Check sheet for the modelled part. Datum: model origin and axes. Units: mm. A direction names the side the tool comes from. Round coordinates to 2 decimals unless told otherwise and drop trailing zeros. Loops run counter-clockwise (first coordinate to the right, second up) from the corner with the lowest first, then second, coordinate; pieces in that order, holes last. Notation, with made-up numbers: (-8.5, 55.25) -> (12.5, 55.25) arc R13 ccw to (12.5, 76.25) -> close; hole circle Ø3 at (10, -6.5). An arc over 180 degrees is marked (long way). Return JSON: item names as keys, results as strings.
from build123d import *

# Parameters (mm, degrees)
SKETCH2_R           = 66.04
BOSS_EXTRUDE1_DEPTH = 19.05
FILLET1_R           = 0.635
SKETCH4_W           = 12.7
SKETCH4_H           = 9.0994385
SKETCH4_W_2         = 9.0994385
SKETCH4_H_2         = 12.7
CUT_EXTRUDE2_DEPTH  = 96.317709267
SKETCH5_W           = 52.324
SKETCH5_H           = 19.05
CUT_EXTRUDE3_DEPTH  = 17.272


with BuildPart() as part:
    # Sketch2 → Boss-Extrude1 (new body)
    with BuildSketch(Plane(origin=(0, 0, 0), x_dir=(1, 0, 0), z_dir=(0, 1, 0))):
        with Locations(Location((0, 0, 0), (0, 0, 90))):
            Circle(SKETCH2_R)
    extrude(amount=BOSS_EXTRUDE1_DEPTH)

    # Fillet1
    fillet1_edges = [part.edges().sort_by_distance(p)[0] for p in [
        (0, 0, 66.04),
        (0, 19.05, 66.04),
    ]]
    fillet(fillet1_edges, radius=FILLET1_R)

    # Sketch4 → Cut-Extrude2 (cut, through all)
    with BuildSketch(Plane.XZ):
        with Locations((0, -65.50971925)):
            Rectangle(SKETCH4_W, SKETCH4_H)
        with Locations((-65.50971925, 0)):
            Rectangle(SKETCH4_W_2, SKETCH4_H_2)
        with Locations((0, 65.50971925)):
            Rectangle(SKETCH4_W, SKETCH4_H)
        with Locations((65.50971925, 0)):
            Rectangle(SKETCH4_W_2, SKETCH4_H_2)
    extrude(amount=-CUT_EXTRUDE2_DEPTH, mode=Mode.SUBTRACT)

    # Sketch5 → Cut-Extrude3 (cut)
    with BuildSketch(Plane(origin=(0, 19.05, 0), x_dir=(1, 0, 0), z_dir=(0, 1, 0))):
        Rectangle(SKETCH5_W, SKETCH5_H)
    extrude(amount=-CUT_EXTRUDE3_DEPTH, mode=Mode.SUBTRACT)


solid = part.part
Q1. Go/stop test with flat-tipped pins: pin 1 (2 mm diameter, centred on x = -43.5, y = 8, fed in from +Z); pin 2 (1.4 mm diameter, centred on x = 62, y = 10, fed in from -Z); pin 3 (5 mm diameter, centred on x = 17.5, z = -27, fed in from -Y); pin 4 (8.5 mm diameter, centred on y = 12.5, z = -4, fed in from +X). Record where each tip stops, or that it passes through.
Results list:
{"pin 1": "z = 50.55", "pin 2": "z = -24.57", "pin 3": "y = 0", "pin 4": "x = 65.73"}
Q2. Draft check along Z on faces 1 (the flat face through (-6.35, 9, -63)), 2 (the cylindrical face through (47.15, 9.4, -46.24)), 3 (the flat face through (-63, 9, 6.35)), 4 (the cylindrical face through (46.24, 9.4, 47.15)). Enter one of: released by +Z, released by -Z, zero draft, split by the parting line, or undercut.
Results list:
{"face 1": "zero draft", "face 2": "released by -Z", "face 3": "undercut", "face 4": "released by +Z"}
Q3. Tool access check on faces 5 (the flat face through (0, 9, -60.96)), 6 (the flat face through (60.96, 9, 0)), 7 (the flat face through (0, 9, 60.96)). Record the directions out of +Z, -Z, +X, -X, +Y, -Y that give a thin tool (end or side, any length) a straight path to the whole face; none if there is none.
Results list:
{"face 5": "-Z, +Y, -Y", "face 6": "+X, +Y, -Y", "face 7": "+Z, +Y, -Y"}
Q4. Section check A-A (y = 14). Record the boundary of the cut face in (x, z) (3 decimals), then the cut area to 3 significant figures.
Results list:
{"outline": "(-65.734, -6.35) arc R66.04 ccw to (-6.35, -65.734) -> (-6.35, -60.96) -> (6.35, -60.96) -> (6.35, -65.734) arc R66.04 ccw to (65.734, -6.35) -> (60.96, -6.35) -> (60.96, 6.35) -> (65.734, 6.35) arc R66.04 ccw to (6.35, 65.734) -> (6.35, 60.96) -> (-6.35, 60.96) -> (-6.35, 65.734) arc R66.04 ccw to (-65.734, 6.35) -> (-60.96, 6.35) -> (-60.96, -6.35) -> close; hole (-26.162, -9.525) -> (26.162, -9.525) -> (26.162, 9.525) -> (-26.162, 9.525) -> close", "area": "12,500 mm^2"}
Q5. Material ranges on line 1 (Z direction, x = -1, y = 15.5) (3 decimals); line 2 (X direction, y = 7.25, z = 3.5); line 3 (Y direction, x = -10, z = 4), recorded low to high.
Results list:
{"line 1": "-60.96 to -9.525, 9.525 to 60.96", "line 2": "-60.96 to -26.16, 26.16 to 60.96", "line 3": "0 to 1.78"}
Q6. Section check B-B (z = 4.5). Record the boundary of the cut face in (x, y), then the cut area to 3 significant figures.
Results list:
{"outline": "(-60.96, 0) -> (60.96, 0) -> (60.96, 19.05) -> (26.16, 19.05) -> (26.16, 1.78) -> (-26.16, 1.78) -> (-26.16, 19.05) -> (-60.96, 19.05) -> close", "area": "1,420 mm^2"}
